The model under review builds one solid part; all positions refer to its coordinate system, in mm. A direction names the side the tool comes from. Give positions to 0.01 mm unless a question says otherwise; leave off trailing zeros. Loops run counter-clockwise (first coordinate to the right, second up) from the corner with the lowest first, then second, coordinate; pieces in that order, holes last. Notation, with made-up numbers: (14, 58) - (36, 58) arc R15 ccw to (36, 73) - close; hole circle Ø8 at (-31.5, -18.75). An arc over 180 degrees is marked (long way). Answer as a JSON object with one key per item and string values.
from build123d import *

# Parameters (mm, degrees)
SKETCH1_R           = 6.1
BOSS_EXTRUDE1_DEPTH = 25
SKETCH2_W           = 160
SKETCH2_H           = 30
CUT_EXTRUDE1_DEPTH  = 50
CUT_EXTRUDE5_DEPTH  = 30
CUT_EXTRUDE7_DEPTH  = 30
FILLET3_R           = 10
SKETCH8_R           = 3
CUT_EXTRUDE8_DEPTH  = 20
SKETCH9_R           = 3.15
CUT_EXTRUDE9_DEPTH  = 4
SKETCH10_R          = 3.5
CUT_EXTRUDE10_DEPTH = 3
SKETCH11_R          = 6.5
CUT_EXTRUDE11_DEPTH = 5
CUT_EXTRUDE12_START = -5
SKETCH12_R          = 6.5
CUT_EXTRUDE12_DEPTH = 5


with BuildPart() as part:
    # Sketch1 → Boss-Extrude1 (new, symmetric)
    with BuildSketch(Plane.XY):
        with BuildLine():
            Line((-110, -15), (110, -15))
            ThreePointArc((110, -15), (125, 0), (110, 15))
            Line((110, 15), (-110, 15))
            ThreePointArc((-110, 15), (-125, 0), (-110, -15))
        make_face()
        with Locations((-90, 0)):
            Circle(SKETCH1_R, mode=Mode.SUBTRACT)
        with Locations((90, 0)):
            Circle(SKETCH1_R, mode=Mode.SUBTRACT)
    extrude(amount=BOSS_EXTRUDE1_DEPTH, both=True)

    # Sketch2 → Cut-Extrude1 (cut)
    with BuildSketch(Plane(origin=(0, 15, 0), x_dir=(1, 0, 0), z_dir=(0, 1, 0))):
        with Locations((-125, 0)):
            Rectangle(SKETCH2_W, SKETCH2_H)
    extrude(amount=-CUT_EXTRUDE1_DEPTH, mode=Mode.SUBTRACT)

    # Sketch4 → Cut-Extrude5 (cut)
    with BuildSketch(Plane.XY.offset(15)):
        Polygon((-45, 15), (-45, 0), (-15, 15), align=None)
    extrude(amount=-CUT_EXTRUDE5_DEPTH, mode=Mode.SUBTRACT)

    # Sketch7 → Cut-Extrude7 (cut)
    with BuildSketch(Plane(origin=(0, 0, 15), x_dir=(-1, 0, 0), z_dir=(0, 0, -1))):
        Polygon((45, 0), (45, -15), (15, -15), align=None)
    extrude(amount=CUT_EXTRUDE7_DEPTH, mode=Mode.SUBTRACT)

    # Fillet3
    fillet3_edges = [part.edges().sort_by_distance(p)[0] for p in [
        (-45, 0, 0),
    ]]
    fillet(fillet3_edges, radius=FILLET3_R)

    # Sketch8 → Cut-Extrude8 (cut)
    with BuildSketch(Plane.XY.offset(25)):
        with Locations((-12.5, 8.5)):
            Circle(SKETCH8_R)
        with Locations((2.5, 8.5)):
            Circle(SKETCH8_R)
        with Locations(Location((2.5, -8.5, 0), (0, 0, 180))):
            Circle(SKETCH8_R)
        with Locations(Location((-12.5, -8.5, 0), (0, 0, 180))):
            Circle(SKETCH8_R)
    extrude(amount=-CUT_EXTRUDE8_DEPTH, mode=Mode.SUBTRACT)

    # Sketch9 → Cut-Extrude9 (cut)
    with BuildSketch(Plane.XY.offset(25)):
        with Locations((-72, 0)):
            Circle(SKETCH9_R)
        with Locations((-54, 0)):
            Circle(SKETCH9_R)
    extrude(amount=-CUT_EXTRUDE9_DEPTH, mode=Mode.SUBTRACT)

    # Sketch10 → Cut-Extrude10 (cut)
    with BuildSketch(Plane.XY.offset(25)):
        with Locations((-72, 0)):
            Circle(SKETCH10_R)
        with Locations((-54, 0)):
            Circle(SKETCH10_R)
    extrude(amount=-CUT_EXTRUDE10_DEPTH, mode=Mode.SUBTRACT)

    # Sketch11 → Cut-Extrude11 (cut)
    with BuildSketch(Plane(origin=(0, 0, 15), x_dir=(-1, 0, 0), z_dir=(0, 0, -1))):
        with Locations((90, 0)):
            Circle(SKETCH11_R)
    extrude(amount=-CUT_EXTRUDE11_DEPTH, mode=Mode.SUBTRACT)

    # Sketch12 → Cut-Extrude12 (cut)
    with BuildSketch(Plane.XY.offset(-15).offset(CUT_EXTRUDE12_START)):
        with Locations(Location((-90, 0, 0), (0, 0, 180))):
            Circle(SKETCH12_R)
    extrude(amount=CUT_EXTRUDE12_DEPTH, mode=Mode.SUBTRACT)


solid = part.part
Q1. For faces 5 (the face through (-84.365, -2.336, -22.535)), 6 (the face through (2, 9, 5)), list the 3-axis set-ups (+Z, -Z, +X, -X, +Y, -Y) from which the entire face can be reached by the end or side of a thin tool; tool diameter is ignored.
Results:
{"face 5": "+Z, -Z", "face 6": "+Z"}
Q2. The part is to be moulded in two halves that separate along Y. For faces 1 (the face through (-32.64, -0.15, -0.21)), 2 (the face through (-12, -9, 5)), 3 (the face through (-9.5, -8.6, 15.1)), 4 (the face through (26, 15, 0)), say which applies: +Y half, -Y half, draft (parallel to the pull), parting line (faces both ways), or undercut.
Results:
{"face 1": "parting line", "face 2": "undercut", "face 3": "undercut", "face 4": "+Y half"}
Q3. Consider section D-D, the plane z = 17.5. State the section outline as (x, y) points, plus the area to 3 significant figures.
Results:
{"outline": "(-110, -15) - (110, -15) arc R15 ccw to (110, 15) - (-110, 15) arc R15 ccw to start; hole circle Ø13 at (-90, 0); hole circle Ø6 at (-12.5, -8.5); hole circle Ø6 at (-12.5, 8.5); hole circle Ø6 at (2.5, -8.5); hole circle Ø6 at (2.5, 8.5); hole circle Ø12.2 at (90, 0)", "area": "6,940 mm^2"}
Q4. Clearance check with flat-ended pins moving along their axes: pin 1 Ø12 at (y, z) = (8, -6) entering from -X; pin 2 Ø5 at (y, z) = (0.5, -8.5) entering from -X; pin 3 Ø12 at (y, z) = (10, -11) entering from -X. State where each tip first meets the part, or that it passes through.
Results:
{"pin 1": "stops at x = -32.44", "pin 2": "stops at x = -32.64", "pin 3": "stops at x = -123.94"}
Q5. Consider section C-C, the plane x = -42.5. State the section outline as (y, z) points.
Results:
{"outline": "(-15, -25) - (15, -25) - (15, -15) - (-15, -15) - close; (-15, 15) - (15, 15) - (15, 25) - (-15, 25) - close"}
Q6. To check wall thickness, follow probe 1 along Y at (x, z) = (-12.5, 13.5); probe 2 along Z at (x, y) = (-51.5, -3.5); probe 3 along Z at (x, y) = (-52, 1). State the ranges of each line that lie inside material, in increasing order. Write a range as [from, to].
Results:
{"probe 1": "y = [-15, -11.5], [-5.5, 5.5], [11.5, 15]", "probe 2": "z = [-25, -15], [15, 25]", "probe 3": "z = [-25, -15], [15, 21]"}
Q7. Consider section B-B, the plane z = -2. State the section outline as (x, y) points.
Results:
{"outline": "(-27.11, -8.94) - (-15, -15) - (110, -15) arc R15 ccw to (110, 15) - (-15, 15) - (-27.11, 8.94) arc R10 ccw to start; hole circle Ø12.2 at (90, 0)"}
Q8. Consider section A-A, the plane x = -90. State the section outline as (y, z) points, plus the area to 3 significant figures.
Results:
{"outline": "(-15, -25) - (-6.1, -25) - (-6.1, -20) - (-6.5, -20) - (-6.5, -15) - (-15, -15) - close; (-15, 15) - (-6.5, 15) - (-6.5, 20) - (-6.1, 20) - (-6.1, 25) - (-15, 25) - close; (6.1, -25) - (15, -25) - (15, -15) - (6.5, -15) - (6.5, -20) - (6.1, -20) - close; (6.1, 20) - (6.5, 20) - (6.5, 15) - (15, 15) - (15, 25) - (6.1, 25) - close", "area": "348 mm^2"}
